from build123d import *

# Parameters (mm, degrees)
BOSS_EXTRUDE1_DEPTH = 50.8
SKETCH3_R           = 1.27
CUT_EXTRUDE2_DEPTH  = 50.8
CUT_EXTRUDE1_DEPTH  = 50.8
CUT_EXTRUDE6_DEPTH  = 50.8
BOSS_EXTRUDE3_DEPTH = 20.32
SKETCH4_W           = 10.16
SKETCH4_H           = 15.24
CUT_EXTRUDE3_DEPTH  = 50.8
SKETCH5_R           = 2.54
CUT_EXTRUDE5_DEPTH  = 50.8
SKETCH8_R           = 2.54
BOSS_EXTRUDE2_DEPTH = 2.54
LPATTERN1_COUNT     = 2
LPATTERN1_PITCH     = 12.7
CUT_EXTRUDE7_DEPTH  = 20.32
SKETCH12_W          = 5.08
SKETCH12_H          = 19.941398178
CUT_EXTRUDE8_DEPTH  = 21.59
CUT_EXTRUDE9_DEPTH  = 5.08
LPATTERN2_COUNT     = 2
LPATTERN2_PITCH     = 15.24
CUT_EXTRUDE10_DEPTH = 40.767
SKETCH14_R          = 7.638081415
BOSS_EXTRUDE4_DEPTH = 2.54
SKETCH16_R          = 2.54
BOSS_EXTRUDE5_DEPTH = 2.54
SKETCH21_W          = 3.776239755
SKETCH21_H          = 7.410355269
CUT_EXTRUDE14_DEPTH = 2.54
CUT_EXTRUDE15_DEPTH = 9.906
SKETCH23_R          = 2.7
CUT_EXTRUDE16_DEPTH = 4.2
FILLET1_R           = 0.254
SKETCH24_R          = 1.7526
CUT_EXTRUDE17_DEPTH = 5.47


with BuildPart() as part:
    # Sketch1 → Boss-Extrude1 (new body)
    with BuildSketch(Plane(origin=(0, 0, 0), x_dir=(1, 0, 0), z_dir=(0, 1, 0))):
        with BuildLine():
            Line((-20.32, 27.095319289), (-20.32, 11.855319289))
            ThreePointArc((-20.32, 11.855319289), (-19.204076836, 9.161242453), (-16.51, 8.045319289))
            Line((-16.51, 8.045319289), (-3.81, 8.045319289))
            ThreePointArc((-3.81, 8.045319289), (-1.115923164, 9.161242453), (0, 11.855319289))
            Line((0, 11.855319289), (0, 27.095319289))
            ThreePointArc((0, 27.095319289), (-1.115923164, 29.789396126), (-3.81, 30.905319289))
            Line((-3.81, 30.905319289), (-16.51, 30.905319289))
            ThreePointArc((-16.51, 30.905319289), (-19.204076836, 29.789396126), (-20.32, 27.095319289))
        make_face()
    extrude(amount=BOSS_EXTRUDE1_DEPTH)

    # Sketch3 → Cut-Extrude2 (cut)
    with BuildSketch(Plane(origin=(0, 50.8, 0), x_dir=(1, 0, 0), z_dir=(0, 1, 0))):
        with Locations(Location((-10.16, 10.585319289, 0), (0, 0, 270))):
            Circle(SKETCH3_R)
        with Locations(Location((-10.16, 28.365319289, 0), (0, 0, 270))):
            Circle(SKETCH3_R)
    extrude(amount=-CUT_EXTRUDE2_DEPTH, mode=Mode.SUBTRACT)

    # Sketch2 → Cut-Extrude1 (cut)
    with BuildSketch(Plane.ZY.offset(20.32)):
        with BuildLine():
            Line((-27.095319289, 7.62), (-30.905319289, 15.24))
            Line((-30.905319289, 15.24), (-30.905319289, -5.08))
            Line((-30.905319289, -5.08), (-8.045319289, -5.08))
            Line((-8.045319289, -5.08), (-8.045319289, 15.24))
            Line((-8.045319289, 15.24), (-11.855319289, 7.62))
            ThreePointArc((-11.855319289, 7.62), (-19.475319289, 0), (-27.095319289, 7.62))
        make_face()
        with BuildLine():
            Line((-11.821559044, 42.970355269), (-8.045319289, 35.56))
            Line((-8.045319289, 35.56), (-8.045319289, 55.88))
            Line((-8.045319289, 55.88), (-30.905319289, 55.88))
            Line((-30.905319289, 55.88), (-30.905319289, 35.56))
            Line((-30.905319289, 35.56), (-27.092422036, 42.951560486))
            ThreePointArc((-27.092422036, 42.951560486), (-19.46663852, 50.799994215), (-11.821559044, 42.970355269))
        make_face()
    extrude(amount=-CUT_EXTRUDE1_DEPTH, mode=Mode.SUBTRACT)

    # Sketch7 → Cut-Extrude6 (cut)
    with BuildSketch(Plane.XY.offset(-8.045319289)):
        Polygon((-15.24, 50.8), (-12.7, 50.8), (-12.7, 35.56), (-7.62, 35.56), (-7.62, 50.8), (-5.08, 50.8), (-5.08, 35.56), (0, 35.56), (0, 59.156438057), (-20.32, 59.156438057), (-20.32, 35.56), (-15.24, 35.56), align=None)
    extrude(amount=-CUT_EXTRUDE6_DEPTH, mode=Mode.SUBTRACT)

    # Sketch9 → Boss-Extrude3 (add)
    with BuildSketch(Plane.ZY.offset(20.32)):
        with BuildLine():
            Line((-19.475319289, 35.56), (-30.961107471, 35.56))
            Line((-30.961107471, 35.56), (-30.961107471, 45.935432902))
            ThreePointArc((-30.961107471, 45.935432902), (-30.291229548, 47.014503778), (-29.026975399, 46.892882091))
            Line((-29.026975399, 46.892882091), (-27.092843326, 42.985764183))
            ThreePointArc((-27.092843326, 42.985764183), (-24.794356941, 37.723605727), (-19.475319289, 35.56))
        make_face()
    extrude(amount=-BOSS_EXTRUDE3_DEPTH)

    # Sketch4 → Cut-Extrude3 (cut)
    with BuildSketch(Plane.XY.offset(-8.045319289)):
        with Locations((-10.16, 7.62)):
            Rectangle(SKETCH4_W, SKETCH4_H)
    extrude(amount=-CUT_EXTRUDE3_DEPTH, mode=Mode.SUBTRACT)

    # Sketch5 → Cut-Extrude5 (cut)
    with BuildSketch(Plane.ZY.offset(20.32)):
        with Locations((-19.475319289, 7.62)):
            Circle(SKETCH5_R)
    extrude(amount=-CUT_EXTRUDE5_DEPTH, mode=Mode.SUBTRACT)

    # Sketch8 → Boss-Extrude2 (add)
    with BuildSketch(Plane.ZY.offset(15.24)):
        with Locations(Location((-19.441559044, 43.179995622, 0), (0, 0, 180))):
            Circle(SKETCH8_R)
    boss_extrude2 = extrude(amount=BOSS_EXTRUDE2_DEPTH)

    # LPattern1: Boss-Extrude2 ×2
    with Locations(*[(i * LPATTERN1_PITCH, 0, 0) for i in range(1, LPATTERN1_COUNT)]):
        add(boss_extrude2)

    # Sketch10 → Cut-Extrude7 (cut)
    with BuildSketch(Plane.XZ.offset(-35.56)):
        with BuildLine():
            Line((-16.51, -30.905319289), (-3.81, -30.905319289))
            ThreePointArc((-3.81, -30.905319289), (-1.115923164, -29.789396126), (0, -27.095319289))
            Line((0, -27.095319289), (5.770912039, -37.258829719))
            Line((5.770912039, -37.258829719), (-26.797758959, -37.890739908))
            Line((-26.797758959, -37.890739908), (-20.32, -27.095319289))
            ThreePointArc((-20.32, -27.095319289), (-19.204076836, -29.789396126), (-16.51, -30.905319289))
        make_face()
    extrude(amount=-CUT_EXTRUDE7_DEPTH, mode=Mode.SUBTRACT)

    # Sketch12 → Cut-Extrude8 (cut)
    with BuildSketch(Plane.XY.offset(-8.045319289)):
        with Locations((-10.16, 45.530699089)):
            Rectangle(SKETCH12_W, SKETCH12_H)
    extrude(amount=-CUT_EXTRUDE8_DEPTH, mode=Mode.SUBTRACT)

    # Sketch13 → Cut-Extrude9 (cut)
    with BuildSketch(Plane.ZY.offset(20.32)):
        Polygon((-19.475319289, 35.56), (-8.045319289, 30.82545932), (-1.320705488, 30.82545932), (-1.320705488, 35.56), align=None)
    cut_extrude9 = extrude(amount=-CUT_EXTRUDE9_DEPTH, mode=Mode.SUBTRACT)

    # LPattern2: Cut-Extrude9 ×2
    with Locations(*[(i * LPATTERN2_PITCH, 0, 0) for i in range(1, LPATTERN2_COUNT)]):
        add(cut_extrude9, mode=Mode.SUBTRACT)

    # Sketch15 → Cut-Extrude10 (cut, symmetric)
    with BuildSketch(Plane(origin=(0, 35.56, 0), x_dir=(1, 0, 0), z_dir=(0, 1, 0))):
        with BuildLine():
            Line((-10.16, 25.825319289), (-10.16, 13.125319289))
            ThreePointArc((-10.16, 13.125319289), (-7.62, 10.585319289), (-10.16, 8.045319289))
            Line((-10.16, 8.045319289), (12.124662948, -15.989120413))
            Line((12.124662948, -15.989120413), (8.97204404, 40.385502166))
            Line((8.97204404, 40.385502166), (-10.16, 30.905319289))
            ThreePointArc((-10.16, 30.905319289), (-12.7, 28.365319289), (-10.16, 25.825319289))
        make_face()
    extrude(amount=CUT_EXTRUDE10_DEPTH, both=True, mode=Mode.SUBTRACT)

    # Sketch14 → Boss-Extrude4 (add)
    with BuildSketch(Plane(origin=(-12.7, 0, 0), x_dir=(0, 0, -1), z_dir=(1, 0, 0))):
        with Locations((19.457237874, 43.161918585)):
            Circle(SKETCH14_R)
    extrude(amount=BOSS_EXTRUDE4_DEPTH)

    # Sketch16 → Boss-Extrude5 (add)
    with BuildSketch(Plane(origin=(-10.16, 0, 0), x_dir=(0, 0, -1), z_dir=(1, 0, 0))):
        with Locations(Location((19.457237874, 43.161918585, 0), (0, 0, 180))):
            Circle(SKETCH16_R)
    extrude(amount=BOSS_EXTRUDE5_DEPTH)

    # Sketch21 → Cut-Extrude14 (cut)
    with BuildSketch(Plane.ZY.offset(15.24)):
        with Locations((-9.933439167, 39.265177635)):
            Rectangle(SKETCH21_W, SKETCH21_H)
    extrude(amount=-CUT_EXTRUDE14_DEPTH, mode=Mode.SUBTRACT)

    # Sketch22 → Cut-Extrude15 (cut)
    with BuildSketch(Plane.ZY.offset(15.24)):
        Polygon((-8.045319289, 30.82545932), (-11.821559044, 32.38965536), (-11.821559044, 35.56), (-8.045319289, 35.56), align=None)
    extrude(amount=-CUT_EXTRUDE15_DEPTH, mode=Mode.SUBTRACT)

    # Sketch23 → Cut-Extrude16 (cut)
    with BuildSketch(Plane(origin=(-10.16, 0, 0), x_dir=(0, 0, -1), z_dir=(1, 0, 0))):
        with Locations((19.475319289, 22.86)):
            Circle(SKETCH23_R)
    extrude(amount=-CUT_EXTRUDE16_DEPTH, mode=Mode.SUBTRACT)

    # Fillet1
    fillet1_edges = [part.edges().sort_by_distance(p)[0] for p in [
        (-10.16, 22.86, -16.775319289),
    ]]
    fillet(fillet1_edges, radius=FILLET1_R)

    # Sketch24 → Cut-Extrude17 (cut)
    with BuildSketch(Plane(origin=(-14.36, 0, 0), x_dir=(0, 0, -1), z_dir=(1, 0, 0))):
        with Locations((19.475319289, 22.86)):
            Circle(SKETCH24_R)
    extrude(amount=-CUT_EXTRUDE17_DEPTH, mode=Mode.SUBTRACT)


solid = part.part
CAD build for the part. Positions are in the model's coordinates, mm. A direction names the side the tool comes from. Coordinates: 2 decimals unless noted, no trailing zeros. Write each loop counter-clockwise with the first axis right and the second up, starting at its lowest first coordinate (ties: lowest second). Pieces come first, ordered by that corner, then holes. Notation, with made-up numbers: M 45,62 L 69,62 A6 cw 69,68 Z; hole C 14.5,-21.75 d6. An arc over 180 degrees is marked long. Return JSON: item names as keys, results as strings.
Item 1: Slice it at A-A, the plane x = -16. Write the cut outline in (y, z).
Findings below:
{"outline": "M 7.62,-27.1 L 15.24,-30.91 L 46.3,-30.91 A1.2 ccw 46.89,-29.03 L 42.99,-27.09 A7.62 cw 35.56,-19.48 L 30.83,-8.05 L 15.24,-8.05 L 7.62,-11.86 A7.62 ccw Z; C 43.18,-19.44 d5.08; hole C 7.62,-19.48 d5.08; hole C 22.86,-19.48 d3.51"}
Item 2: Two-plate mould, pull along Z, no slides. Class faces 5 (the cylindrical face through (-16.49, 41.04, -20.81)), 6 (the flat face through (-20.32, 17, -19)), 7 (the flat face through (-13, 31, -30.905)): +Z half, -Z half, draft (parallel to the pull), parting line (faces both ways), or undercut.
Findings below:
{"face 5": "undercut", "face 6": "draft", "face 7": "-Z half"}
Item 3: Which spindle directions (+Z, -Z, +X, -X, +Y, -Y) get a long thin tool onto all of the face, cutting with end or side? Do faces 1 (the flat face through (-17.78, 43, -19)), 2 (the flat face through (-12, 15.24, -17)), 3 (the flat face through (-9, 34, -11.822)), 4 (the flat face through (-19.83, 23, -19)). Say none if no direction does.
Findings below:
{"face 1": "+Z, -X, +Y", "face 2": "+Z, -Z, +X, -Y", "face 3": "+Z, +X, -X, +Y", "face 4": "+X"}
Item 4: Drop flat-ended pins along their axis: pin 1 Ø6 at (x, z) = (-10, -23.5) entering from -Y; pin 2 Ø2 at (y, z) = (39.5, -26.5) entering from +X; pin 3 Ø5 at (x, z) = (-9, -16) entering from +Y. Give the stop position or say it passes through.
Findings below:
{"pin 1": "stops at y = 15.24", "pin 2": "stops at x = -10.16", "pin 3": "stops at y = 50.7"}
Item 5: Slice it at D-D, the plane y = 40. Write the cut outline in (x, z), and give its area (3 significant figures).
Findings below:
{"outline": "M -20.32,-27.1 A3.81 ccw -16.51,-30.91 L -10.16,-30.91 A2.54 cw -12.36,-29.64 L -12.7,-29.64 L -12.7,-26.41 L -10.16,-26.41 L -10.16,-12.5 L -12.7,-12.5 L -12.7,-11.82 L -15.24,-11.82 L -15.24,-26.4 L -20.32,-26.4 Z", "area": "105 mm2"}
Item 6: Slice it at B-B, the plane y = 22.86. Write the cut outline in (x, z).
Findings below:
{"outline": "M -20.32,-27.1 A3.81 ccw -16.51,-30.91 L -10.16,-30.91 A2.54 cw -10.16,-25.83 L -10.16,-22.43 A0.25 ccw -10.41,-22.18 L -14.36,-22.18 L -14.36,-21.23 L -19.83,-21.23 L -19.83,-17.72 L -14.36,-17.72 L -14.36,-16.78 L -10.41,-16.78 A0.25 ccw -10.16,-16.52 L -10.16,-13.13 A2.54 ccw -10.16,-8.05 L -16.51,-8.05 A3.81 ccw -20.32,-11.86 Z; hole C -10.16,-10.59 d2.54"}
Item 7: Slice it at C-C, the plane z = -14.75. Write the cut outline in (x, y), and give its area (3 significant figures).
Findings below:
{"outline": "M -20.32,1.64 L -15.24,1.64 L -15.24,15.24 L -10.16,15.24 L -10.16,35.56 L -12.7,35.56 L -12.7,37.15 L -10.16,37.15 L -10.16,49.18 L -15.24,49.18 L -15.24,33.6 L -20.32,33.6 Z", "area": "331 mm2"}
Item 8: Probe line 1 (Y direction, x = -12.25, z = -17.25); line 2 (X direction, y = 18, z = -21); line 3 (Y direction, x = -11.25, z = -21.5). List the from-to ranges inside material, lowest first. Write a range as from..to.
Findings below:
{"line 1": "y = 15.24..21.33, 24.39..35.56, 35.85..50.47", "line 2": "x = -20.32..-10.16", "line 3": "y = 15.24..21.07, 24.65..35.56, 35.8..50.52"}
